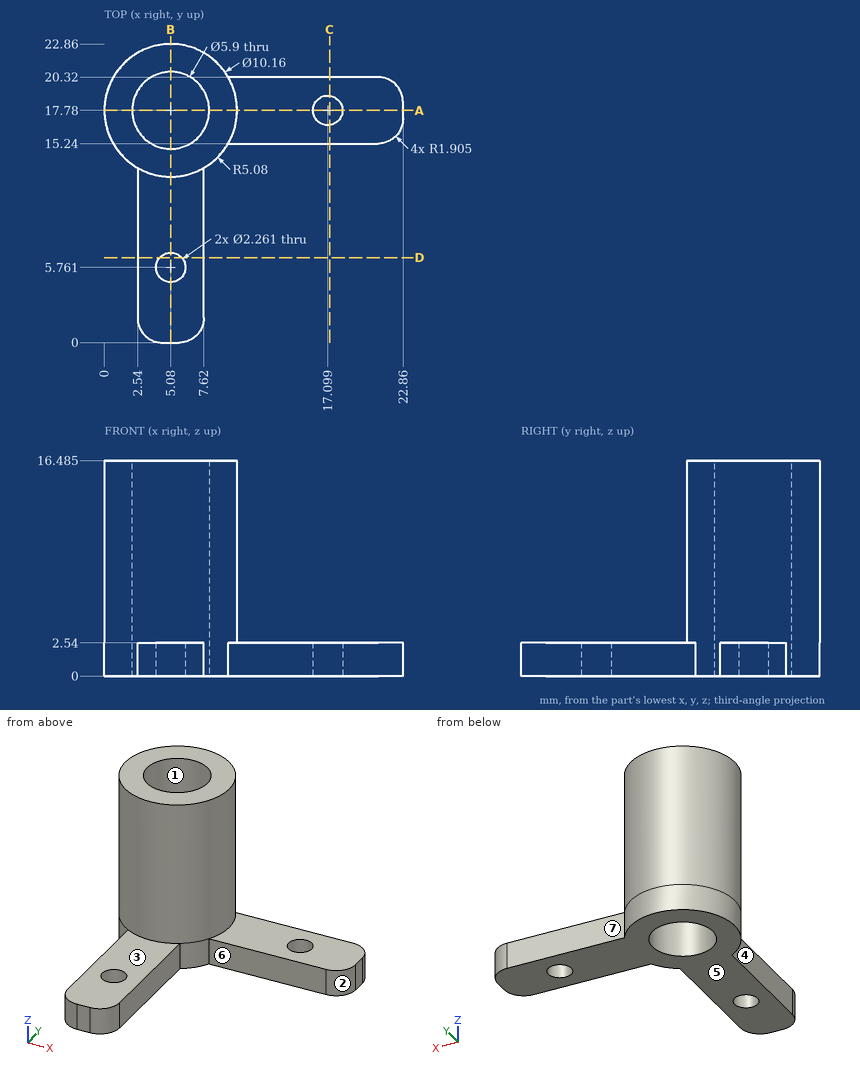
Geometry: see drawing. Coordinates: mm, zero at the bounding-box minimum. A direction names the side the tool comes from. Coordinates: 2 decimals unless noted, no trailing zeros. Write each loop counter-clockwise with the first axis right and the second up, starting at its lowest first coordinate (ties: lowest second). Pieces come first, ordered by that corner, then holes.
1) Material intervals for line 1 along Y through (x, z) = (5.08, 1.4); line 2 along Y through (x, z) = (5.08, 8); line 3 along X through (y, z) = (4.5, 1.5), sorted ascending.
2) Section C-C on x = 17.25. Output: boundary loops of the cut face in (y, z).
3) Set-up query: the marked faces 4, 5, 6 and 7. Return all of +Z, -Z, +X, -X, +Y, -Y with unobstructed straight access to the full face (end or side cutting, diameter ignored); none if empty.
4) Pin query (flat end, axial travel): pin 1 Ø5 at (y, z) = (16, 2) entering from +X; pin 2 Ø3 at (x, z) = (15.5, 1.5) entering from -Y; pin 3 Ø4.5 at (x, y) = (5.08, 17.78) entering from +Z; pin 4 Ø3 at (y, z) = (6, 1) entering from +X. Return the tip coordinate at first contact, or that it passes through.
5) Section B-B on x = 5.08. Output: boundary loops of the cut face in (y, z) (1 decimal).
6) Mould query, pull axis Y, two halves, no side actions, for the marked faces 1, 2 and 3. Classes: pulls with the +Y half, pulls with the -Y half, needs draft (parallel to the pull), parting line crosses it, or undercut.
7) Section A-A on y = 17.78. Output: boundary loops of the cut face in (x, z) (1 decimal).
8) Section D-D on y = 6.5. Output: boundary loops of the cut face in (x, z) (1 decimal).
Check result:
1. line 1: y = 0 to 4.63, 6.89 to 14.83, 20.73 to 22.86
1. line 2: y = 12.7 to 14.83, 20.73 to 22.86
1. line 3: x = 2.54 to 7.62
2. outline: (15.24, 0) - (16.66, 0) - (16.66, 2.54) - (15.24, 2.54) - close; (18.9, 0) - (20.32, 0) - (20.32, 2.54) - (18.9, 2.54) - close
3. face 4: +Z, -Z, -X, -Y
3. face 5: -Z, +X, -X, +Y, -Y
3. face 6: +Z, -Z, +X, -Y
3. face 7: +Z, -Z, +X, +Y
4. pin 1: stops at x = 22.86
4. pin 2: stops at y = 15.24
4. pin 3: passes through
4. pin 4: stops at x = 7.62
5. outline: (0, 0) - (4.6, 0) - (4.6, 2.5) - (0, 2.5) - close; (6.9, 0) - (14.8, 0) - (14.8, 16.5) - (12.7, 16.5) - (12.7, 2.5) - (6.9, 2.5) - close; (20.7, 0) - (22.9, 0) - (22.9, 16.5) - (20.7, 16.5) - close
6. face 1: undercut
6. face 2: pulls with the -Y half
6. face 3: needs draft
7. outline: (0, 0) - (2.1, 0) - (2.1, 16.5) - (0, 16.5) - close; (8, 0) - (16, 0) - (16, 2.5) - (10.2, 2.5) - (10.2, 16.5) - (8, 16.5) - close; (18.2, 0) - (22.9, 0) - (22.9, 2.5) - (18.2, 2.5) - close
8. outline: (2.5, 0) - (4.2, 0) - (4.2, 2.5) - (2.5, 2.5) - close; (5.9, 0) - (7.6, 0) - (7.6, 2.5) - (5.9, 2.5) - close
